Can you work these out from the model? Positions are in its coordinate system, mm. A direction names the side the tool comes from. Coordinates: 2 decimals unless noted, no trailing zeros. Order: outer loops, then holes, each group sorted by start corner. A loop starts at its lowest first (then second) coordinate and runs counter-clockwise, first axis right, second up. Notation, with made-up numbers: (28.5, 63) -> (85.5, 63) arc R24 ccw to (85.5, 82) -> close; hole circle Ø11 at (14, 78). An arc over 180 degrees is marked (long way). Use a Markdown table: item, result. Add a question column.
1. If I drill on line 1 along Y through (x, z) = (0, 18.5); line 2 along X through (y, z) = (8, 23.5); line 3 along X through (y, z) = (7.5, 8), over which ranges is the centre line in solid material (lowest first)? Write a range as from..to.
2. We'd pull the mould along X, two halves only. Please class faces 4 (the flat face through (130, -26, 15)), 5 (the cylindrical face through (105, 0, 15)), 6 (the flat face through (71, -16, 30)), 7 (the cylindrical face through (-20, 0, 15)): pulls with the +X half, pulls with the -X half, needs draft (parallel to the pull), parting line crosses it, or undercut.
3. For pin 1 Ø15 at (x, z) = (30, 10) entering from -Y; pin 2 Ø16 at (x, y) = (115, 0) entering from +Z; pin 3 Ø8 at (x, z) = (115.5, 18.5) entering from -Y; pin 4 Ø6 at (x, y) = (12, -2.5) entering from -Z, each with a flat end and sliding along its axis, tell me the tip position at first contact or that it passes through.
4. Suppose I cut it at B-B, the plane z = 3. List the corners of the cut face in (x, y) for me.
5. Suppose I cut it at A-A, the plane y = 0. List the corners of the cut face in (x, z) for me, then the cut area to 3 significant figures.
6. Suppose I cut it at C-C, the plane x = 115. List the corners of the cut face in (y, z) for me, then the cut area to 3 significant figures.
7. Suppose I cut it at D-D, the plane y = -46. List the corners of the cut face in (x, z) for me.
8. For faces 1 (the cylindrical face through (107.19, -55.21, 16.73)), 2 (the flat face through (66, 20, 15)), 3 (the flat face through (49, -20, 15)), which set-ups out of +Z, -Z, +X, -X, +Y, -Y let a thin tool reach every point of the face, with its end or its side?
```python
from build123d import *

# Parameters (mm, degrees)
BOSS_EXTRUDE1_DEPTH = 30
SKETCH2_R           = 8
CUT_EXTRUDE1_DEPTH  = 30
SKETCH3_R           = 10
CUT_EXTRUDE2_DEPTH  = 30


with BuildPart() as part:
    # Sketch1 → Boss-Extrude1 (new body)
    with BuildSketch(Plane(origin=(0, 0, 0), x_dir=(0, 1, 0), z_dir=(0, 0, 1))):
        with BuildLine():
            Line((-20, 0), (-20, -100))
            Line((-20, -100), (-70, -100))
            Line((-70, -100), (-70, -130))
            Line((-70, -130), (20, -130))
            Line((20, -130), (20, 0))
            ThreePointArc((20, 0), (0, 20), (-20, 0))
        make_face()
    extrude(amount=BOSS_EXTRUDE1_DEPTH)

    # Sketch2 → Cut-Extrude1 (cut)
    with BuildSketch(Plane.XZ.offset(70)):
        with Locations(Location((115, 15, 0), (0, 0, 270))):
            Circle(SKETCH2_R)
    extrude(amount=-CUT_EXTRUDE1_DEPTH, mode=Mode.SUBTRACT)

    # Sketch3 → Cut-Extrude2 (cut)
    with BuildSketch(Plane.XY.offset(30)):
        Circle(SKETCH3_R)
        with Locations((115, 0)):
            Circle(SKETCH3_R)
    extrude(amount=-CUT_EXTRUDE2_DEPTH, mode=Mode.SUBTRACT)


solid = part.part
```
Worked out:
| question | item | result |
|---|---|---|
| 1 | line 1 | y = -20..-10, 10..20 |
| 1 | line 2 | x = -18.33..-6, 6..109, 121..130 |
| 1 | line 3 | x = -18.54..-6.61, 6.61..108.39, 121.61..130 |
| 2 | face 4 | pulls with the +X half |
| 2 | face 5 | undercut |
| 2 | face 6 | needs draft |
| 2 | face 7 | pulls with the -X half |
| 3 | pin 1 | stops at y = -20 |
| 3 | pin 2 | passes through |
| 3 | pin 3 | stops at y = -40 |
| 3 | pin 4 | stops at z = 0 |
| 4 | outline | (0, -20) -> (100, -20) -> (100, -70) -> (130, -70) -> (130, 20) -> (0, 20) arc R20 ccw to start; hole circle Ø20 at (0, 0); hole circle Ø20 at (115, 0) |
| 5 | outline | (-20, 0) -> (-10, 0) -> (-10, 30) -> (-20, 30) -> close; (10, 0) -> (105, 0) -> (105, 30) -> (10, 30) -> close; (125, 0) -> (130, 0) -> (130, 30) -> (125, 30) -> close |
| 5 | area | 3,300 mm² |
| 6 | outline | (-70, 0) -> (-10, 0) -> (-10, 30) -> (-70, 30) -> (-70, 23) -> (-40, 23) -> (-40, 7) -> (-70, 7) -> close; (10, 0) -> (20, 0) -> (20, 30) -> (10, 30) -> close |
| 6 | area | 1,620 mm² |
| 7 | outline | (100, 0) -> (130, 0) -> (130, 30) -> (100, 30) -> close; hole circle Ø16 at (115, 15) |
| 8 | face 1 | -Y |
| 8 | face 2 | +Z, -Z, +X, -X, +Y |
| 8 | face 3 | +Z, -Z, -X, -Y |
